```python
from build123d import *

# Parameters (mm, degrees)
PAD007_DEPTH = 12.8
SKETCH026_R  = 3.05
PAD008_DEPTH = 5.2
SKETCH027_R  = 3.05
PAD009_DEPTH = 5.2
SKETCH028_R  = 3.05
PAD010_DEPTH = 5.2


with BuildPart() as part:
    # Sketch025 → Pad007 (new body)
    with BuildSketch(Plane.XY):
        with BuildLine():
            Line((64.9839392466, -187.2), (9, -187.2))
            Line((9, -187.2), (9, -200))
            Line((9, -200), (64.9839392466, -200))
            ThreePointArc((64.9839392466, -200), (129.9678784932, -178.8854382), (170.1301616704, -123.60679775))
            Line((187.4301503097, -70.3629075216), (170.1301616704, -123.60679775))
            Line((187.4301503097, -70.3629075216), (175.2566269011, -66.4074899936))
            Line((157.9566382618, -119.651380222), (175.2566269011, -66.4074899936))
            ThreePointArc((64.9839392466, -187.2), (122.4442272638, -168.530020672), (157.9566382618, -119.651380222))
        make_face()
    extrude(amount=PAD007_DEPTH)

    # Sketch026 (on Face9 of Pad007) → Pad008 (join)
    with BuildSketch(Plane(origin=(0, 0, 0), x_dir=(1, 0, 0), z_dir=(0, 0, -1))):
        with Locations((21.8, 193.6)):
            Circle(SKETCH026_R)
    extrude(amount=PAD008_DEPTH)

    # Sketch027 (on Face4 of Pad008) → Pad009 (join)
    with BuildSketch(Plane(origin=(0, 0, 0), x_dir=(1, 0, 0), z_dir=(0, 0, -1))):
        with Locations((126.2060528785, 173.707729436)):
            Circle(SKETCH027_R)
    extrude(amount=PAD009_DEPTH)

    # Sketch028 (on Face4 of Pad009) → Pad010 (join)
    with BuildSketch(Plane(origin=(0, 0, 0), x_dir=(1, 0, 0), z_dir=(0, 0, -1))):
        with Locations((177.3879710774, 80.5587221662)):
            Circle(SKETCH028_R)
    extrude(amount=PAD010_DEPTH)


solid = part.part
```
Geometry: final body of the model. Coordinates: model frame, mm. A direction names the side the tool comes from. Coordinates: 2 decimals unless noted, no trailing zeros. Order: outer loops, then holes, each group sorted by start corner. A loop starts at its lowest first (then second) coordinate and runs counter-clockwise, first axis right, second up. Notation, with made-up numbers: (8.5, 2.5) -> (16.5, 2.5) arc R31 ccw to (16.5, 31.5) -> close; hole circle Ø4 at (13, 62). An arc over 180 degrees is marked (long way). Write item = value, one per line.
(1) Cut plane D-D on x = 155. Return loops of the section in (y, z).
Solved:
outline = (-153.63, 0) -> (-127.57, 0) -> (-127.57, 12.8) -> (-153.63, 12.8) -> close
(2) Cut plane B-B on x = 21.8. Return loops of the section in (y, z).
Solved:
outline = (-200, 0) -> (-196.65, 0) -> (-196.65, -5.2) -> (-190.55, -5.2) -> (-190.55, 0) -> (-187.2, 0) -> (-187.2, 12.8) -> (-200, 12.8) -> close
(3) Pin query (flat end, axial travel): pin 1 Ø4 at (x, z) = (45, 7.5) entering from +Y; pin 2 Ø2 at (x, z) = (113, 3.5) entering from -Y; pin 3 Ø10 at (x, z) = (129.5, 7.5) entering from -Y. Return the tip coordinate at first contact, or that it passes through.
Solved:
pin_1 = -187.2
pin_2 = -189.5
pin_3 = -182.61
(4) Line query: line 1 (Y direction, x = 19, z = 10.5); line 2 (Z direction, x = 167.5, y = -98.5); line 3 (Y direction, x = 106, z = 5). Output: solid intervals per line, ascending.
Solved:
line_1 = -200 to -187.2
line_2 = 0 to 12.8
line_3 = -192.11 to -178.18
(5) Access query for faces 1 (the cylindrical face through (21.403, -196.624, -2.564)), 2 (the flat face through (37, -187.2, 6)), 3 (the flat face through (178.9, -96.61, 6.31)). Directions: +Z, -Z, +X, -X, +Y, -Y. A direction counts if a zero-diameter tool reaches every point of the face in a straight line with its end or side. Return the directions, or none.
Solved:
face_1 = -Z
face_2 = +Z, -Z, -X, +Y
face_3 = +Z, -Z, +X, -Y
(6) Cut plane A-A on z = 4.25. Return loops of the section in (x, y).
Solved:
outline = (9, -200) -> (64.98, -200) arc R110.56 ccw to (170.13, -123.61) -> (187.43, -70.36) -> (175.26, -66.41) -> (157.96, -119.65) arc R97.76 cw to (64.98, -187.2) -> (9, -187.2) -> close
(7) Cut plane C-C on y = -184. Return loops of the section in (x, z).
Solved:
outline = (89.79, 0) -> (122.27, 0) -> (122.27, 12.8) -> (89.79, 12.8) -> close
